Design review of the part built by this model. Coordinates are the model's own, in mm. A direction names the side the tool comes from. Coordinates: 2 decimals unless noted, no trailing zeros. Write each loop counter-clockwise with the first axis right and the second up, starting at its lowest first coordinate (ties: lowest second). Pieces come first, ordered by that corner, then holes.
Q1. For probe 1 along X at (y, z) = (22.5, 4.5) (3 decimals); probe 2 along Y at (x, z) = (95.25, 7); probe 3 along X at (y, z) = (21.5, 5.75) (3 decimals), list the stretches that pass through material, from the lowest coordinate up.
Q2. Machinability: for faces 3 (the flat face through (-122.555, 27, 6)), 4 (the flat face through (47.625, -12, 6)), 5 (the flat face through (48, 0, 5.08)), which of the approach directions +Z, -Z, +X, -X, +Y, -Y give a long, thin tool a straight path to every point of the face, cutting with its end or side? Answer none if there is none.
Q3. Mouldability with a two-part tool opening along X and no side actions: class faces 1 (the conical face through (57.17, 0.22, 12.56)), 2 (the cylindrical face through (80.355, 30.077, 7.542)) as pulls with the +X half, pulls with the -X half, needs draft (parallel to the pull), parting line crosses it, or undercut.
Q4. Take a section at B-B (y = 0). State how many separate pieces and enclosed holes the cut face has, and give its area (3 significant figures).
Q5. Take a section at A-A (x = -12.7). Give the boundary of the cut face in (y, z), and give its area (3 significant figures).
Q6. Insertion check: pin 1 (10.5 mm diameter, centred on x = 81, y = 16, fed in from -Z); pin 2 (8 mm diameter, centred on x = -22, y = 20.5, fed in from -Z); pin 3 (10.5 mm diameter, centred on x = 12.7, y = 0, fed in from +Z); pin 4 (1.5 mm diameter, centred on x = -82, z = 10.5, fed in from +Y). Each pin has a flat end and moves straight along its axis. Give the tip position at first contact, or say it passes through.
```python
from build123d import *

# Parameters (mm, degrees)
SKETCH1_R           = 3.175
SKETCH1_R_2         = 1.7
SKETCH1_R_3         = 1.85
BOSS_EXTRUDE1_DEPTH = 12.7
SKETCH2_R           = 6.6
CUT_EXTRUDE1_DEPTH  = 5.08
FILLET1_R           = 6.35
SKETCH3_R           = 3.175
CUT_EXTRUDE2_DEPTH  = 325.374
SKETCH4_R           = 6.6
CUT_EXTRUDE3_DEPTH  = 12.7
CHAMFER1_SIZE       = 0.5


with BuildPart() as part:
    # Sketch1 → Boss-Extrude1 (new body)
    with BuildSketch(Plane.XY):
        with BuildLine():
            Line((-122.555, 19.05), (-107.315, 19.05))
            Line((-107.315, 19.05), (-107.315, 39.37))
            Line((-107.315, 39.37), (-99.695, 39.37))
            Line((-99.695, 39.37), (-99.695, 19.05))
            Line((-99.695, 19.05), (-86.868, 19.05))
            Line((-86.868, 19.05), (-86.868, 29.21))
            ThreePointArc((-86.868, 29.21), (-86.124051224, 31.006051224), (-84.328, 31.75))
            Line((-84.328, 31.75), (-76.2, 31.75))
            ThreePointArc((-76.2, 31.75), (-74.403948776, 31.006051224), (-73.66, 29.21))
            Line((-73.66, 29.21), (-73.66, 19.05))
            Line((-73.66, 19.05), (73.66, 19.05))
            Line((73.66, 19.05), (73.66, 29.21))
            ThreePointArc((73.66, 29.21), (74.403948776, 31.006051224), (76.2, 31.75))
            Line((76.2, 31.75), (84.328, 31.75))
            ThreePointArc((84.328, 31.75), (86.124051224, 31.006051224), (86.868, 29.21))
            Line((86.868, 29.21), (86.868, 19.05))
            Line((86.868, 19.05), (99.695, 19.05))
            Line((99.695, 19.05), (99.695, 39.37))
            Line((99.695, 39.37), (107.315, 39.37))
            Line((107.315, 39.37), (107.315, 19.05))
            Line((107.315, 19.05), (122.555, 19.05))
            Line((122.555, 19.05), (122.555, 39.37))
            Line((122.555, 39.37), (130.175, 39.37))
            Line((130.175, 39.37), (130.175, 19.05))
            Line((130.175, 19.05), (130.175, -19.05))
            Line((130.175, -19.05), (-130.175, -19.05))
            Line((-130.175, -19.05), (-130.175, 19.05))
            Line((-130.175, 19.05), (-130.175, 39.37))
            Line((-130.175, 39.37), (-122.555, 39.37))
            Line((-122.555, 39.37), (-122.555, 19.05))
        make_face()
        with Locations((-117.475, 0)):
            Circle(SKETCH1_R, mode=Mode.SUBTRACT)
        with Locations(Location((117.475, 0, 0), (0, 0, 180))):
            Circle(SKETCH1_R, mode=Mode.SUBTRACT)
        with Locations((-80.264, 27.94)):
            Circle(SKETCH1_R_2, mode=Mode.SUBTRACT)
        with Locations((-80.264, 8.89)):
            Circle(SKETCH1_R_2, mode=Mode.SUBTRACT)
        with Locations(Location((80.264, 8.89, 0), (0, 0, 180))):
            Circle(SKETCH1_R_2, mode=Mode.SUBTRACT)
        with Locations(Location((80.264, 27.94, 0), (0, 0, 180))):
            Circle(SKETCH1_R_2, mode=Mode.SUBTRACT)
        with Locations((-95.25, 12.7)):
            Circle(SKETCH1_R_3, mode=Mode.SUBTRACT)
        with Locations(Location((-95.25, -7.62, 0), (0, 0, 180))):
            Circle(SKETCH1_R_3, mode=Mode.SUBTRACT)
        with Locations((95.25, -7.62)):
            Circle(SKETCH1_R_3, mode=Mode.SUBTRACT)
        with Locations(Location((95.25, 12.7, 0), (0, 0, 180))):
            Circle(SKETCH1_R_3, mode=Mode.SUBTRACT)
    extrude(amount=BOSS_EXTRUDE1_DEPTH)

    # Sketch2 → Cut-Extrude1 (cut)
    with BuildSketch(Plane(origin=(0, 0, 0), x_dir=(-1, 0, 0), z_dir=(0, 0, -1))):
        with Locations((-47.625, 0)):
            Circle(SKETCH2_R)
        with Locations(Location((47.625, 0, 0), (0, 0, 180))):
            Circle(SKETCH2_R)
        with BuildLine():
            Line((-73.66, 29.21), (-73.66, 19.05))
            Line((-73.66, 19.05), (-73.66, -19.05))
            Line((-73.66, -19.05), (-86.868, -19.05))
            Line((-86.868, -19.05), (-86.868, 19.05))
            Line((-86.868, 19.05), (-86.868, 29.21))
            ThreePointArc((-86.868, 29.21), (-86.124051224, 31.006051224), (-84.328, 31.75))
            Line((-84.328, 31.75), (-76.2, 31.75))
            ThreePointArc((-76.2, 31.75), (-74.403948776, 31.006051224), (-73.66, 29.21))
        make_face()
        with BuildLine():
            Line((73.66, -19.05), (73.66, 19.05))
            Line((73.66, 19.05), (73.66, 29.21))
            ThreePointArc((73.66, 29.21), (74.403948776, 31.006051224), (76.2, 31.75))
            Line((76.2, 31.75), (84.328, 31.75))
            ThreePointArc((84.328, 31.75), (86.124051224, 31.006051224), (86.868, 29.21))
            Line((86.868, 29.21), (86.868, 19.05))
            Line((86.868, 19.05), (86.868, -19.05))
            Line((86.868, -19.05), (73.66, -19.05))
        make_face()
    extrude(amount=-CUT_EXTRUDE1_DEPTH, mode=Mode.SUBTRACT)

    # Fillet1
    fillet1_edges = [part.edges().sort_by_distance(p)[0] for p in [
        (-126.365, 39.37, 0),
        (-126.365, 39.37, 12.7),
        (-103.505, 39.37, 12.7),
        (-103.505, 39.37, 0),
        (103.505, 39.37, 0),
        (103.505, 39.37, 12.7),
        (126.365, 39.37, 12.7),
        (126.365, 39.37, 0),
    ]]
    fillet(fillet1_edges, radius=FILLET1_R - 0.0001)  # a hair under: the kernel refuses the full size

    # Sketch3 → Cut-Extrude2 (cut)
    with BuildSketch(Plane(origin=(130.175, 0, 0), x_dir=(0, 0, -1), z_dir=(1, 0, 0))):
        with Locations(Location((-6.35, 33.02, 0), (0, 0, 90))):
            Circle(SKETCH3_R)
    extrude(amount=-CUT_EXTRUDE2_DEPTH, mode=Mode.SUBTRACT)

    # Sketch4 → Cut-Extrude3 (cut)
    with BuildSketch(Plane.XY.offset(12.7)):
        with Locations((12.7, 0)):
            Circle(SKETCH4_R)
        with Locations(Location((-12.7, 0, 0), (0, 0, 180))):
            Circle(SKETCH4_R)
        with BuildLine():
            Line((47.625, 14.22), (47.625, 9.91))
            ThreePointArc((47.625, 9.91), (57.535, 0), (47.625, -9.91))
            Line((47.625, -9.91), (47.625, -14.22))
            ThreePointArc((47.625, -14.22), (61.845, 0), (47.625, 14.22))
        make_face()
        with BuildLine():
            Line((-47.625, -9.91), (-47.625, -14.22))
            ThreePointArc((-47.625, -14.22), (-61.845, 0), (-47.625, 14.22))
            Line((-47.625, 14.22), (-47.625, 9.91))
            ThreePointArc((-47.625, 9.91), (-57.535, 0), (-47.625, -9.91))
        make_face()
    extrude(amount=-CUT_EXTRUDE3_DEPTH, mode=Mode.SUBTRACT)

    # Chamfer1
    chamfer1_edges = [part.edges().sort_by_distance(p)[0] for p in [
        (-97.1, 12.7, 12.7),
        (-114.935, 19.05, 12.7),
        (93.4, -7.62, 12.7),
        (-122.555, 26.03505, 12.7),
        (97.1, 12.7, 12.7),
        (0, -19.05, 12.7),
        (-130.175, 6.98505, 0),
        (-130.175, 6.98505, 12.7),
        (-130.175, 37.51015735, 10.84015735),
        (-130.175, 37.51015735, 1.85984265),
        (-107.315, 26.03505, 0),
        (-122.555, 37.51015735, 10.84015735),
        (-122.555, 37.51015735, 1.85984265),
        (122.555, 26.03505, 12.7),
        (99.695, 26.03505, 12.7),
        (-107.315, 26.03505, 12.7),
        (-107.315, 37.51015735, 1.85984265),
        (-107.315, 37.51015735, 10.84015735),
        (-99.695, 37.51015735, 1.85984265),
        (-99.695, 37.51015735, 10.84015735),
        (114.935, 19.05, 12.7),
        (99.695, 26.03505, 0),
        (99.695, 37.51015735, 10.84015735),
        (99.695, 37.51015735, 1.85984265),
        (122.555, 26.03505, 0),
        (107.315, 37.51015735, 10.84015735),
        (107.315, 37.51015735, 1.85984265),
        (122.555, 37.51015735, 1.85984265),
        (122.555, 37.51015735, 10.84015735),
        (130.175, 37.51015735, 1.85984265),
        (130.175, 37.51015735, 10.84015735),
        (107.315, 26.03505, 12.7),
        (57.535, 0, 12.7),
        (47.625, -12.065, 12.7),
        (61.845, 0, 12.7),
        (47.625, 12.065, 12.7),
        (-57.535, 0, 12.7),
        (-47.625, 12.065, 12.7),
        (-61.845, 0, 12.7),
        (-47.625, -12.065, 12.7),
        (-6.1, 0, 12.7),
        (6.1, 0, 12.7),
        (-122.555, 26.03505, 0),
        (-99.695, 26.03505, 0),
        (93.2815, 19.05, 12.7),
        (107.315, 26.03505, 0),
        (130.175, 6.98505, 0),
        (86.868, 24.13, 12.7),
        (86.124051224, 31.006051224, 12.7),
        (80.264, 31.75, 12.7),
        (130.175, 6.98505, 12.7),
        (74.403948776, 31.006051224, 12.7),
        (73.66, 24.13, 12.7),
        (0, 19.05, 12.7),
        (-73.66, 24.13, 12.7),
        (-74.403948776, 31.006051224, 12.7),
        (-80.264, 31.75, 12.7),
        (-120.65, 0, 12.7),
        (-86.124051224, 31.006051224, 12.7),
        (120.65, 0, 12.7),
        (-86.868, 24.13, 12.7),
        (-81.964, 27.94, 12.7),
        (-93.2815, 19.05, 12.7),
        (-81.964, 8.89, 12.7),
        (81.964, 8.89, 12.7),
        (-99.695, 26.03505, 12.7),
        (81.964, 27.94, 12.7),
        (-93.4, -7.62, 12.7),
    ]]
    chamfer(chamfer1_edges, length=CHAMFER1_SIZE)


solid = part.part
```
Response:
1. probe 1: x = -130.175 to -122.555, -107.315 to -99.695, 99.695 to 107.315, 122.555 to 130.175
1. probe 2: y = -19.05 to -9.47, -5.77 to 10.85, 14.55 to 19.05
1. probe 3: x = -130.175 to -122.555, -107.315 to -99.695, -86.868 to -73.66, 73.66 to 86.868, 99.695 to 107.315, 122.555 to 130.175
2. face 3: +Z, -Z, +Y
2. face 4: +Z, -Z
2. face 5: -Z
3. face 1: undercut
3. face 2: needs draft
4. separate pieces: 7
4. enclosed holes: 0
4. area: 2,430 mm2
5. outline: (-19.05, 0) - (-6.6, 0) - (-6.6, 12.2) - (-7.1, 12.7) - (-18.55, 12.7) - (-19.05, 12.2) - close; (6.6, 0) - (19.05, 0) - (19.05, 12.2) - (18.55, 12.7) - (7.1, 12.7) - (6.6, 12.2) - close
5. area: 316 mm2
6. pin 1: stops at z = 5.08
6. pin 2: stops at z = 0
6. pin 3: passes through
6. pin 4: stops at y = 31.75
